The listing builds one solid part. Answer for the finished solid, in the listing's coordinates (mm). A direction names the side the tool comes from. Give positions to 0.01 mm unless a question says otherwise; leave off trailing zeros. Write each loop counter-clockwise with the first axis right and the second up, starting at its lowest first coordinate (ties: lowest second). Pieces come first, ordered by that corner, then holes. Notation, with made-up numbers: (69.5, 29) - (124.5, 29) arc R25 ccw to (124.5, 56) - close; hole circle Ø10 at (17.5, -13.75). An arc over 180 degrees is marked (long way). Answer in a Markdown table with one row per item. Add a question column.
from build123d import *

# Parameters (mm, degrees)
DODANIE_WYCI_GNI_CIE1_DEPTH = 12
DODANIE_WYCI_GNI_CIE2_DEPTH = 2
WYTNIJ_WYCI_GNI_CIE1_REACH  = 27.507
SZKIC3_R                    = 1.75
ZAOKR_GLENIE1_R             = 7.5


with BuildPart() as part:
    # Szkic1 → Dodanie-wyciągnięcie1 (new, symmetric)
    with BuildSketch(Plane.XY):
        with BuildLine():
            ThreePointArc((-10.6, 0), (0, 10.6), (10.6, 0))
            Line((10.6, 0), (18.5, 0))
            Line((18.5, 0), (18.5, -5.9))
            Line((18.5, -5.9), (7.6, -5.9))
            Line((7.6, -5.9), (7.6, 0))
            ThreePointArc((7.6, 0), (0, 7.6), (-7.6, 0))
            Line((-7.6, 0), (-7.6, -5.9))
            Line((-7.6, -5.9), (-18.5, -5.9))
            Line((-18.5, -5.9), (-18.5, 0))
            Line((-18.5, 0), (-10.6, 0))
        make_face()
    extrude(amount=DODANIE_WYCI_GNI_CIE1_DEPTH, both=True)

    # Szkic2 → Dodanie-wyciągnięcie2 (add)
    with BuildSketch(Plane(origin=(0, 0, -12), x_dir=(-1, 0, 0), z_dir=(0, 0, -1))):
        with BuildLine():
            Line((18.5, 0), (10.6, 0))
            ThreePointArc((10.6, 0), (0, 10.6), (-10.6, 0))
            Line((-10.6, 0), (-18.5, 0))
            Line((-18.5, 0), (-18.5, -5.9))
            Line((-18.5, -5.9), (-7.6, -5.9))
            Line((-7.6, -5.9), (-7.6, 0))
            ThreePointArc((-7.6, 0), (0, 7.6), (7.6, 0))
            Line((7.6, 0), (7.6, -5.9))
            Line((7.6, -5.9), (18.5, -5.9))
            Line((18.5, -5.9), (18.5, 0))
        make_face()
        with BuildLine():
            ThreePointArc((4.6, 0), (0, 4.6), (-4.6, 0))
            Line((-4.6, 0), (-4.6, -5.9))
            Line((-4.6, -5.9), (-7.6, -5.9))
            Line((-7.6, -5.9), (-7.6, 0))
            ThreePointArc((-7.6, 0), (0, 7.6), (7.6, 0))
            Line((7.6, 0), (7.6, -5.9))
            Line((7.6, -5.9), (4.6, -5.9))
            Line((4.6, -5.9), (4.6, 0))
        make_face()
    extrude(amount=DODANIE_WYCI_GNI_CIE2_DEPTH)

    # Szkic3 → Wytnij-wyciągnięcie1 (cut, up to next)
    with BuildSketch(Plane(origin=(0, 0, 0), x_dir=(1, 0, 0), z_dir=(0, 1, 0)), mode=Mode.PRIVATE) as wytnij_wyci_gni_cie1_sk1:
        with Locations(Location((-14.5, 0, 0), (0, 0, 270))):
            Circle(SZKIC3_R)
    wytnij_wyci_gni_cie1_tool1 = extrude(wytnij_wyci_gni_cie1_sk1.sketch, amount=-WYTNIJ_WYCI_GNI_CIE1_REACH, mode=Mode.PRIVATE) & part.part
    # Szkic3 → Wytnij-wyciągnięcie1 (cut, up to next)
    with BuildSketch(Plane(origin=(0, 0, 0), x_dir=(1, 0, 0), z_dir=(0, 1, 0)), mode=Mode.PRIVATE) as wytnij_wyci_gni_cie1_sk2:
        with Locations(Location((14.5, 0, 0), (0, 0, 270))):
            Circle(SZKIC3_R)
    wytnij_wyci_gni_cie1_tool2 = extrude(wytnij_wyci_gni_cie1_sk2.sketch, amount=-WYTNIJ_WYCI_GNI_CIE1_REACH, mode=Mode.PRIVATE) & part.part
    add(wytnij_wyci_gni_cie1_tool1.solids().sort_by_distance((-14.5, 0, 0))[0], mode=Mode.SUBTRACT)
    add(wytnij_wyci_gni_cie1_tool2.solids().sort_by_distance((14.5, 0, 0))[0], mode=Mode.SUBTRACT)

    # Zaokrąglenie1
    zaokr_glenie1_edges = [part.edges().sort_by_distance(p)[0] for p in [
        (-18.5, -2.95, 12),
        (18.5, -2.95, 12),
    ]]
    fillet(zaokr_glenie1_edges, radius=ZAOKR_GLENIE1_R)


solid = part.part
1. The mould has two halves that part along X. Classify faces 5 (the face through (18.5, -3, -5)), 6 (the face through (-12.765, -2.909, -0.228)), 7 (the face through (-7.6, -3, 0)), 8 (the face through (1, 8, 12)): +X half, -X half, draft (parallel to the pull), parting line (faces both ways), or undercut.
2. Given pin 1 Ø6.5 at (x, z) = (-15.5, 3.5) entering from +Y; pin 2 Ø3 at (x, z) = (14.5, 0) entering from -Y; pin 3 Ø2 at (x, y) = (4, 2) entering from +Z; pin 4 Ø1 at (x, z) = (-5.5, 8.5) entering from -Y, each flat-ended and moving along its own axis, determine where each tip first touches the part or whether it passes through.
3. Section C-C (z = -4) is taken. Give the vertices of the cut face in (x, y).
4. Section B-B (x = -14.5) is taken. Give the vertices of the cut face in (y, z).
5. Section A-A (z = 0) is taken. Give the vertices of the cut face in (x, y).
6. Section D-D (y = 7) is taken. Give the vertices of the cut face in (x, z).
7. Straight lines are drawn through the part: L1, parallel to X at y = -1.6, z = 0; L2, parallel to X at y = -5, z = -9.25; L3, parallel to X at y = 4.5, z = 8. For each, find the intervals that lie inside material, in ascending order. Write a range as [from, to].
8. A tool of negligible diameter and unlimited length cuts with its end or side. For faces 1 (the face through (0.17, 7.6, 0.17)), 2 (the face through (4.6, -3, -13)), 3 (the face through (12.7, 0, -0.8)), 4 (the face through (12, -5.9, -1)), from which of +Z, -Z, +X, -X, +Y, -Y can it reach the whole face along a straight path? Write none if from no direction.
Geometry check:
| question | item | result |
|---|---|---|
| 1 | face 5 | +X half |
| 1 | face 6 | undercut |
| 1 | face 7 | undercut |
| 1 | face 8 | draft |
| 2 | pin 1 | y = 0 |
| 2 | pin 2 | through |
| 2 | pin 3 | z = -12 |
| 2 | pin 4 | y = 4.66 |
| 3 | outline | (-18.5, -5.9) - (-7.6, -5.9) - (-7.6, 0) arc R7.6 cw to (7.6, 0) - (7.6, -5.9) - (18.5, -5.9) - (18.5, 0) - (10.6, 0) arc R10.6 ccw to (-10.6, 0) - (-18.5, 0) - close |
| 4 | outline | (-5.9, -14) - (0, -14) - (0, -1.75) - (-5.9, -1.75) - close; (-5.9, 1.75) - (0, 1.75) - (0, 11.13) - (-5.9, 11.13) - close |
| 5 | outline | (-18.5, -5.9) - (-16.25, -5.9) - (-16.25, 0) - (-18.5, 0) - close; (-12.75, -5.9) - (-7.6, -5.9) - (-7.6, 0) arc R7.6 cw to (7.6, 0) - (7.6, -5.9) - (12.75, -5.9) - (12.75, 0) - (10.6, 0) arc R10.6 ccw to (-10.6, 0) - (-12.75, 0) - close; (16.25, -5.9) - (18.5, -5.9) - (18.5, 0) - (16.25, 0) - close |
| 6 | outline | (-7.96, -14) - (7.96, -14) - (7.96, 12) - (2.96, 12) - (2.96, -12) - (-2.96, -12) - (-2.96, 12) - (-7.96, 12) - close |
| 7 | L1 | [-18.5, -16.25], [-12.75, -7.6], [7.6, 12.75], [16.25, 18.5] |
| 7 | L2 | [-18.5, -7.6], [7.6, 18.5] |
| 7 | L3 | [-9.6, -6.12], [6.12, 9.6] |
| 8 | face 1 | +Z, -Y |
| 8 | face 2 | +Z, -Z, -Y |
| 8 | face 3 | +Z, -Z, +X, +Y |
| 8 | face 4 | +Z, -Z, +X, -X, -Y |
